Verification items for the finished model (mm, model axes). Give positions to 0.01 mm unless a question says otherwise; leave off trailing zeros. Write each loop counter-clockwise with the first axis right and the second up, starting at its lowest first coordinate (ties: lowest second). Pieces come first, ordered by that corner, then holes. Notation, with made-up numbers: (-9.5, -24) - (40.5, -24) arc R25 ccw to (40.5, 3) - close; hole circle Ø7 at (-7, 14). An arc over 180 degrees is marked (long way). Answer as a JSON object with one key per item and string values. Group by question number.
Item 1: Scan lines: line 1 along X through (y, z) = (8.5, 54.75); line 2 along Z through (x, y) = (-250, 9); line 3 along Z through (x, y) = (287, 6.25). Record each from-to range of solid material in increasing order. Write a range as [from, to].
Item 2: Sectioned sample at C-C, the plane y = 13. Record the boundary of the cut face in (x, z).
Item 3: Sectioned sample at A-A, the plane z = 54.75. Record the boundary of the cut face in (x, y), and give its area (3 significant figures).
Item 4: Sectioned sample at D-D, the plane x = 287.5. Record the boundary of the cut face in (y, z), and give its area (3 significant figures).
Item 5: Sectioned sample at B-B, the plane x = -250. Record the boundary of the cut face in (y, z).
```python
from build123d import *

# Parameters (mm, degrees)
SKETCH1_W                      = 765
SKETCH1_H                      = 374.5
BOSS_EXTRUDE1_DEPTH            = 16
CUT_EXTRUDE1_REACH             = 18
SKETCH2_R                      = 50
CUT_EXTRUDE1_DIRECTION_2_DEPTH = 1


with BuildPart() as part:
    # Sketch1 → Boss-Extrude1 (new body)
    with BuildSketch(Plane(origin=(0, 0, 0), x_dir=(1, 0, 0), z_dir=(0, 1, 0))):
        Rectangle(SKETCH1_W, SKETCH1_H)
    extrude(amount=BOSS_EXTRUDE1_DEPTH)

    # Sketch2 → Cut-Extrude1 (cut, up to next)
    with BuildSketch(Plane(origin=(0, 16, 0), x_dir=(1, 0, 0), z_dir=(0, 1, 0)), mode=Mode.PRIVATE) as cut_extrude1_sk1:
        with Locations((-250, -54.75)):
            Circle(SKETCH2_R)
    cut_extrude1_tool1 = extrude(cut_extrude1_sk1.sketch, amount=-CUT_EXTRUDE1_REACH, mode=Mode.PRIVATE) & part.part
    add(cut_extrude1_tool1.solids().sort_by_distance((-250, 16, 54.75))[0], mode=Mode.SUBTRACT)
    # Sketch2 → Cut-Extrude1 (cut, up to next)
    with BuildSketch(Plane(origin=(0, 16, 0), x_dir=(1, 0, 0), z_dir=(0, 1, 0)), mode=Mode.PRIVATE) as cut_extrude1_sk2:
        with Locations((250, -54.75)):
            Circle(SKETCH2_R)
    cut_extrude1_tool2 = extrude(cut_extrude1_sk2.sketch, amount=-CUT_EXTRUDE1_REACH, mode=Mode.PRIVATE) & part.part
    add(cut_extrude1_tool2.solids().sort_by_distance((250, 16, 54.75))[0], mode=Mode.SUBTRACT)

    # Sketch2 → Cut-Extrude1 direction 2 (cut)
    with BuildSketch(Plane(origin=(0, 16, 0), x_dir=(1, 0, 0), z_dir=(0, 1, 0))):
        with Locations((-250, -54.75)):
            Circle(SKETCH2_R)
        with Locations((250, -54.75)):
            Circle(SKETCH2_R)
    extrude(amount=CUT_EXTRUDE1_DIRECTION_2_DEPTH, mode=Mode.SUBTRACT)


solid = part.part
```
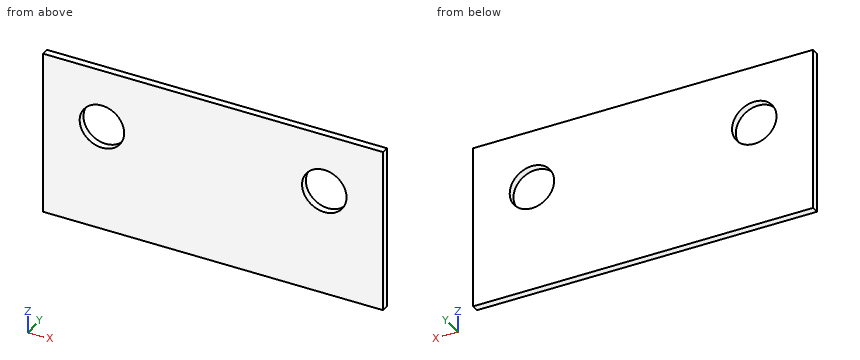
Geometry check:
{
 "1": {"line 1": "[-382.5, -300], [-200, 200], [300, 382.5]", "line 2": "[-187.25, 4.75], [104.75, 187.25]", "line 3": "[-187.25, 21.12], [88.38, 187.25]"},
 "2": {"outline": "(-382.5, -187.25) - (382.5, -187.25) - (382.5, 187.25) - (-382.5, 187.25) - close; hole circle Ø100 at (-250, 54.75); hole circle Ø100 at (250, 54.75)"},
 "3": {"outline": "(-382.5, 0) - (-300, 0) - (-300, 16) - (-382.5, 16) - close; (-200, 0) - (200, 0) - (200, 16) - (-200, 16) - close; (300, 0) - (382.5, 0) - (382.5, 16) - (300, 16) - close", "area": "9,040 mm^2"},
 "4": {"outline": "(0, -187.25) - (16, -187.25) - (16, 21.68) - (0, 21.68) - close; (0, 87.82) - (16, 87.82) - (16, 187.25) - (0, 187.25) - close", "area": "4,930 mm^2"},
 "5": {"outline": "(0, -187.25) - (16, -187.25) - (16, 4.75) - (0, 4.75) - close; (0, 104.75) - (16, 104.75) - (16, 187.25) - (0, 187.25) - close"}
}
